from build123d import *

# Parameters (mm, degrees)
F0_W     = 76.2
F0_H     = 50.8
F1_DEPTH = 127
F2_T     = -2.54
F3_R     = 12.7
F4_DEPTH = 76.201
F6_DEPTH = 76.201
F7_SIZE  = 5.08
F9_DEPTH = 50.8
F9_TAPER = -10
F10_T    = -2.54


with BuildPart() as f1:
    # F0 (on Front) → F1 (new body)
    with BuildSketch(Plane.XZ):
        with Locations((38.1, 25.4)):
            Rectangle(F0_W, F0_H)
    extrude(amount=F1_DEPTH)

    # F2
    f2_openings = [f1.faces().sort_by_distance(p)[0] for p in [
        (38.1, -127, 25.4),
    ]]
    offset(amount=F2_T, openings=f2_openings)

    # F3 (on face) → F4 (cut, through all)
    with BuildSketch(Plane.YZ.offset(76.2)):
        with Locations((-101.4156882687, 25.4)):
            Circle(F3_R)
        with Locations((-63.3156882687, 25.4)):
            Circle(F3_R)
        with Locations((-25.2156882687, 25.4)):
            Circle(F3_R)
    extrude(amount=-F4_DEPTH, mode=Mode.SUBTRACT)

    # F5 (on face) → F6 (cut, through all)
    with BuildSketch(Plane.YZ.offset(76.2)):
        with BuildLine():
            add(Edge.make_bspline(
                [(-114.3024048609, 50.8), (-116.3753766316, 48.2180029007), (-122.7739913645, 38.3634851462), (-120.2785073467, 21.2308461151), (-125.5979944732, 11.4326219351), (-127, 9.4929700746)],
                knots=[0.1809579396, 0.1809579396, 0.1809579396, 0.1809579396, 0.3115506916, 0.6462020469, 0.7356568333, 0.7356568333, 0.7356568333, 0.7356568333], degree=3))
            Line((-114.3024048609, 50.8), (-127, 50.8))
            Line((-127, 50.8), (-127, 9.4929700746))
        make_face()
    extrude(amount=-F6_DEPTH, mode=Mode.SUBTRACT)

    # F7
    f7_edges = [f1.edges().sort_by_distance(p)[0] for p in [
        (2.54, -64.77, 2.54),
        (73.66, -64.77, 2.54),
        (2.54, -59.366962, 48.26),
        (73.66, -59.366962, 48.26),
        (0, -57.151202, 50.8),
        (76.2, -57.151202, 50.8),
        (0, -63.5, 0),
        (76.2, -63.5, 0),
    ]]
    chamfer(f7_edges, length=F7_SIZE)

    # F8 (on face) → F9 (join)
    with BuildSketch(Plane(origin=(0, 0, 0), x_dir=(-1, 0, 0), z_dir=(0, 1, 0))):
        Polygon((0, 45.72), (-5.08, 50.8), (-71.12, 50.8), (-76.2, 45.72), (-76.2, 9.4929700837), (-76.2, 5.08), (-71.12, 0), (-5.08, 0), (0, 5.08), align=None)
    extrude(amount=F9_DEPTH, taper=F9_TAPER)

    # F10
    f10_openings = [f1.faces().sort_by_distance(p)[0] for p in [
        (38.1, 50.8, 25.4),
    ]]
    offset(amount=F10_T, openings=f10_openings, kind=Kind.INTERSECTION)


solid = f1.part
Geometry check sheet. Reference: the model listing, model coordinates, mm. A direction names the side the tool comes from. Round coordinates to 2 decimals unless told otherwise and drop trailing zeros. Order: outer loops, then holes, each group sorted by start corner. A loop starts at its lowest first (then second) coordinate and runs counter-clockwise, first axis right, second up. Notation, with made-up numbers: M 1,60.5 L 41,60.5 A26 cw 41,74.5 Z; hole C 24,-26 d7. An arc over 180 degrees is marked long. Answer in a Markdown table with one row per item. Add a question column.
Item 1: Depth check by flat-ended pin: pin 1 Ø5 at (x, z) = (36.5, 21.5) entering from -Y; pin 2 Ø10 at (y, z) = (-2, 24) entering from +X; pin 3 Ø2 at (x, z) = (23, 35.5) entering from +Y. Enter the tip coordinate at first touch or a pass-through.
Item 2: Sectioned sample at D-D, the plane y = -98.5. Enter the section's corners in (x, z).
Item 3: Set-up check for faces 5 (the face through (2.58, -58.06, 48.3)), 6 (the face through (38, -56, 50.8)), 7 (the face through (73.7, -58.06, 48.22)), 8 (the face through (38, -59, 48.26)), 9 (the face through (76, 31, 50)): record each of +Z, -Z, +X, -X, +Y, -Y from which the full face is reachable in a straight line by a thin tool's end or side.
Item 4: Sectioned sample at B-B, the plane y = -63. Enter the section's corners in (x, z), plus the area to 3 significant figures.
Item 5: Sectioned sample at C-C, the plane z = 25.4. State how many separate pieces and enclosed holes the cut face has, plus the area to 3 significant figures.
Item 6: Draft check along Y on faces 1 (the face through (1.29, -18.39, 36.11)), 2 (the face through (71.08, -61.57, 45.76)), 3 (the face through (-1.982, 25.865, 25.079)), 4 (the face through (74.95, -18.39, 36.11)). Enter one of: released by +Y, released by -Y, zero draft, split by the parting line, or undercut.
Item 7: Material ranges on L1, parallel to Z at x = 40, y = -37; L2, parallel to X at y = -5, z = 17; L3, parallel to Y at x = 57.5, z = 16, recorded low to high. Write a range as [from, to].
Item 8: Sectioned sample at A-A, the plane y = -43.5. Enter the section's corners in (x, z).
Filled in:
| question | item | result |
|---|---|---|
| 1 | pin 1 | stops at y = -2.54 |
| 1 | pin 2 | stops at x = 76.73 |
| 1 | pin 3 | stops at y = 0 |
| 2 | outline | M 0,5.08 L 5.08,0 L 71.12,0 L 76.2,5.08 L 76.2,13.04 L 73.66,13.04 L 73.66,7.62 L 68.58,2.54 L 7.62,2.54 L 2.54,7.62 L 2.54,13.04 L 0,13.04 Z; M 0,37.76 L 2.54,37.76 L 2.54,43.18 L 7.62,48.26 L 68.58,48.26 L 73.66,43.18 L 73.66,37.76 L 76.2,37.76 L 76.2,45.72 L 71.12,50.8 L 5.08,50.8 L 0,45.72 Z |
| 3 | face 5 | +Z, -X, -Y |
| 3 | face 6 | +Z, +X, -X, -Y |
| 3 | face 7 | +Z, +X, -Y |
| 3 | face 8 | -Y |
| 3 | face 9 | +Y |
| 4 | outline | M 0,5.08 L 5.08,0 L 71.12,0 L 76.2,5.08 L 76.2,12.7 L 73.66,12.7 L 73.66,7.62 L 68.58,2.54 L 7.62,2.54 L 2.54,7.62 L 2.54,12.7 L 0,12.7 Z; M 0,38.1 L 2.54,38.1 L 2.54,43.18 L 7.62,48.26 L 68.58,48.26 L 73.66,43.18 L 73.66,38.1 L 76.2,38.1 L 76.2,45.72 L 71.12,50.8 L 5.08,50.8 L 0,45.72 Z |
| 4 | area | 490 mm² |
| 5 | separate pieces | 7 |
| 5 | enclosed holes | 0 |
| 5 | area | 674 mm² |
| 6 | face 1 | undercut |
| 6 | face 2 | zero draft |
| 6 | face 3 | released by +Y |
| 6 | face 4 | undercut |
| 7 | L1 | z = [0, 2.54], [48.26, 50.8] |
| 7 | L2 | x = [0, 2.54], [73.66, 76.2] |
| 7 | L3 | y = [-2.54, 0] |
| 8 | outline | M 0,5.08 L 5.08,0 L 71.12,0 L 76.2,5.08 L 76.2,45.72 L 71.12,50.8 L 5.08,50.8 L 0,45.72 Z; hole M 2.54,7.62 L 7.62,2.54 L 68.58,2.54 L 73.66,7.62 L 73.66,43.18 L 68.58,48.26 L 7.62,48.26 L 2.54,43.18 Z |
